Model file for the job. Use its own axes, mm. A direction names the side the tool comes from. Round coordinates to 2 decimals unless told otherwise and drop trailing zeros. Write each loop counter-clockwise with the first axis right and the second up, starting at its lowest first coordinate (ties: lowest second). Pieces come first, ordered by that corner, then holes.
```python
from build123d import *

# Parameters (mm, degrees)
SKETCH1_R           = 2.45
BOSS_EXTRUDE1_DEPTH = 50
SKETCH1_2_R         = 2.45
BOSS_EXTRUDE2_DEPTH = 50
SKETCH2_W           = 7
SKETCH2_H           = 7
BOSS_EXTRUDE3_DEPTH = 20
SKETCH2_2_W         = 7
SKETCH2_2_H         = 7
BOSS_EXTRUDE4_DEPTH = 20
SKETCH3_R           = 2.45
CUT_EXTRUDE1_DEPTH  = 8


with BuildPart() as part:
    # Sketch1 → Boss-Extrude1 (new body)
    with BuildSketch(Plane(origin=(0, 0, 0), x_dir=(1, 0, 0), z_dir=(0, 1, 0))):
        Circle(SKETCH1_R)
    extrude(amount=BOSS_EXTRUDE1_DEPTH)

    # Sketch1_2 → Boss-Extrude2 (add)
    with BuildSketch(Plane(origin=(0, 0, 0), x_dir=(1, 0, 0), z_dir=(0, 1, 0))):
        Circle(SKETCH1_2_R)
    extrude(amount=-BOSS_EXTRUDE2_DEPTH)

    # Sketch2 → Boss-Extrude3 (add)
    with BuildSketch(Plane(origin=(0, 0, 0), x_dir=(1, 0, 0), z_dir=(0, 1, 0))):
        Rectangle(SKETCH2_W, SKETCH2_H)
    extrude(amount=BOSS_EXTRUDE3_DEPTH)

    # Sketch2_2 → Boss-Extrude4 (add)
    with BuildSketch(Plane(origin=(0, 0, 0), x_dir=(1, 0, 0), z_dir=(0, 1, 0))):
        Rectangle(SKETCH2_2_W, SKETCH2_2_H)
    extrude(amount=-BOSS_EXTRUDE4_DEPTH)

    # Sketch3 → Cut-Extrude1 (cut, through all)
    with BuildSketch(Plane.XY.offset(3.5)):
        Circle(SKETCH3_R)
    extrude(amount=-CUT_EXTRUDE1_DEPTH, mode=Mode.SUBTRACT)


solid = part.part
```
1) Wall check: probe 1 along Y at (x, z) = (0, -1.75); probe 2 along Y at (x, z) = (-0.5, -2.5); probe 3 along Y at (x, z) = (-2.5, -0.25). Give the ranges that are in metal, low to high.
2) Cut at B-B on z = 0. List the corners of the cut face in (x, y), and give its area (3 significant figures).
3) Flat gauge pin, fed straight in: pin 1 Ø4 at (x, y) = (0, -27) entering from +Z. Where does the tip first touch, or does it go through?
4) Cut at D-D on y = 29.5. List the corners of the cut face in (x, z).
5) Cut at C-C on x = 0. List the corners of the cut face in (y, z).
6) Cut at A-A on y = 0. List the corners of the cut face in (x, z).
7) Pull direction X, two halves, no side cores. Call faces 4 (the face through (-0.5, -2.4, 0)), 5 (the face through (3.5, 0, 0)), 6 (the face through (0, 50, 0)), 7 (the face through (-0.5, -34.8, 2.4)): released by +X, released by -X, zero draft, split by the parting line, or undercut.
8) Which spindle directions (+Z, -Z, +X, -X, +Y, -Y) get a long thin tool onto all of the face, cutting with end or side? Do faces 1 (the face through (-2, -20, -2)), 2 (the face through (-0.5, 35.2, 2.4)), 3 (the face through (-3.5, 0, 0)). Say none if no direction does.
Result sheet:
1. probe 1: y = -50 to -2.45, 2.45 to 50
1. probe 2: y = -20 to -2.4, 2.4 to 20
1. probe 3: y = -20 to 20
2. outline: (-3.5, -20) - (-2.45, -20) - (-2.45, -50) - (2.45, -50) - (2.45, -20) - (3.5, -20) - (3.5, 20) - (2.45, 20) - (2.45, 50) - (-2.45, 50) - (-2.45, 20) - (-3.5, 20) - close; hole circle Ø4.9 at (0, 0)
2. area: 555 mm2
3. pin 1: stops at z = 2.45
4. outline: circle Ø4.9 at (0, 0)
5. outline: (-50, -2.45) - (-20, -2.45) - (-20, -3.5) - (-2.45, -3.5) - (-2.45, 3.5) - (-20, 3.5) - (-20, 2.45) - (-50, 2.45) - close; (2.45, -3.5) - (20, -3.5) - (20, -2.45) - (50, -2.45) - (50, 2.45) - (20, 2.45) - (20, 3.5) - (2.45, 3.5) - close
6. outline: (-3.5, -3.5) - (-2.45, -3.5) - (-2.45, 3.5) - (-3.5, 3.5) - close; (2.45, -3.5) - (3.5, -3.5) - (3.5, 3.5) - (2.45, 3.5) - close
7. face 4: undercut
7. face 5: released by +X
7. face 6: zero draft
7. face 7: split by the parting line
8. face 1: -Y
8. face 2: +Y
8. face 3: +Z, -Z, -X, +Y, -Y
